```python
from build123d import *

# Parameters (mm, degrees)
ESQUISSE1_R        = 3
BOSS_EXTRU_1_DEPTH = 5
CONG_2_R           = 0.5
CHANFREIN1_SIZE    = 0.25


with BuildPart() as part:
    # Esquisse1 → Boss.-Extru.1 (new body)
    with BuildSketch(Plane(origin=(0, 0, 0), x_dir=(1, 0, 0), z_dir=(0, 1, 0))):
        Polygon((0, 5.773502692), (-5, 2.886751346), (-5, -2.886751346), (0, -5.773502692), (5, -2.886751346), (5, 2.886751346), align=None)
        Circle(ESQUISSE1_R, mode=Mode.SUBTRACT)
    extrude(amount=BOSS_EXTRU_1_DEPTH)

    # Congé2
    cong_2_edges = [part.edges().sort_by_distance(p)[0] for p in [
        (-5, 5, 0),
        (5, 2.5, -2.886751346),
        (5, 2.5, 2.886751346),
        (0, 2.5, 5.773502692),
        (-5, 2.5, 2.886751346),
        (-5, 2.5, -2.886751346),
        (0, 2.5, -5.773502692),
        (-2.5, 5, 4.330127019),
        (2.5, 5, 4.330127019),
        (5, 5, 0),
        (2.5, 5, -4.330127019),
        (5, 0, 0),
        (2.5, 0, 4.330127019),
        (-2.5, 0, 4.330127019),
        (-2.5, 5, -4.330127019),
        (-5, 0, 0),
        (-2.5, 0, -4.330127019),
        (2.5, 0, -4.330127019),
    ]]
    fillet(cong_2_edges, radius=CONG_2_R)

    # Chanfrein1
    chanfrein1_edges = [part.edges().sort_by_distance(p)[0] for p in [
        (-3, 0, 0),
        (-3, 5, 0),
    ]]
    chamfer(chanfrein1_edges, length=CHANFREIN1_SIZE)


solid = part.part
```
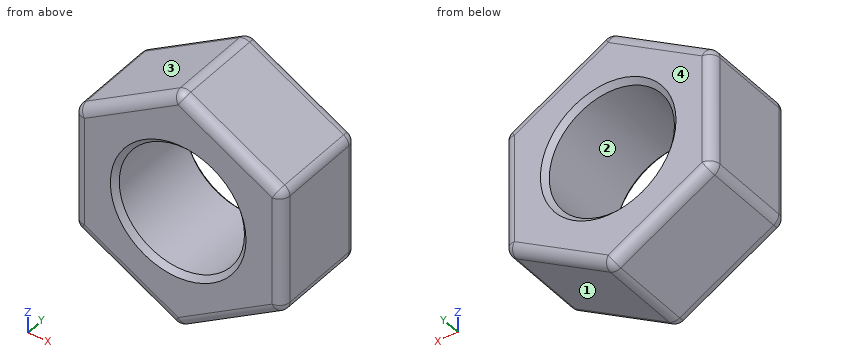
Input: part model. Units: mm. Frame: model coordinates. Face numbers are marked on the shaded views. Coordinates: 2 decimals unless noted, no trailing zeros. Loops run counter-clockwise (first coordinate to the right, second up) from the corner with the lowest first, then second, coordinate; pieces in that order, holes last. Notation, with made-up numbers: M 40.25,20 L 54.25,20 A25 cw 54.25,35 Z; hole C 6.25,42 d10. An arc over 180 degrees is marked long. Use a Markdown table: item, result. Add a question column.
1) Section B-B, the plane y = 2.1. Return the cut outline in (x, z), plus the area to 3 significant figures.
2) Line query: L1, parallel to Z at x = 0, y = 1.3; L2, parallel to X at y = 1.95, z = 0; L3, parallel to X at y = 1.2, z = 0.75. Output: solid intervals per line, ascending. Write a range as from..to.
3) Draft query along X for the marked faces 1, 2, 3 and 4. Return one class per face: +X half, -X half, draft (parallel to the pull), parting line (faces both ways), or undercut.
4) Section A-A, the plane z = 0. Return the cut outline in (x, y).
5) Pin query (flat end, axial travel): P1, Ø2, axis at x = 4, z = -4, coming from the +Y side; P2, Ø2, axis at x = 2.5, y = 3, coming from the +Z side. Return the tip coordinate at first contact, or that it passes through.
Answer below:
| question | item | result |
|---|---|---|
| 1 | outline | M -5,-2.6 A0.5 ccw -4.75,-3.03 L -0.25,-5.63 A0.5 ccw 0.25,-5.63 L 4.75,-3.03 A0.5 ccw 5,-2.6 L 5,2.6 A0.5 ccw 4.75,3.03 L 0.25,5.63 A0.5 ccw -0.25,5.63 L -4.75,3.03 A0.5 ccw -5,2.6 Z; hole C 0,0 d6 |
| 1 | area | 58.2 mm2 |
| 2 | L1 | -5.7..-3, 3..5.7 |
| 2 | L2 | -5..-3, 3..5 |
| 2 | L3 | -5..-2.9, 2.9..5 |
| 3 | face 1 | +X half |
| 3 | face 2 | undercut |
| 3 | face 3 | -X half |
| 3 | face 4 | draft |
| 4 | outline | M -5,0.5 A0.5 ccw -4.5,0 L -3.25,0 L -3,0.25 L -3,4.75 L -3.25,5 L -4.5,5 A0.5 ccw -5,4.5 Z; M 3,0.25 L 3.25,0 L 4.5,0 A0.5 ccw 5,0.5 L 5,4.5 A0.5 ccw 4.5,5 L 3.25,5 L 3,4.75 Z |
| 5 | P1 | y = 5 |
| 5 | P2 | z = 4.91 |
